Geometry check sheet. Reference: the model listing, model coordinates, mm. A direction names the side the tool comes from. Round coordinates to 2 decimals unless told otherwise and drop trailing zeros.
```python
from build123d import *

# Parameters (mm, degrees)
SKETCH1_R           = 2.5
BOSS_EXTRUDE1_DEPTH = 300
FILLET1_R           = 1.47
SKETCH2_R           = 1.5
CUT_EXTRUDE1_DEPTH  = 301.488285961
SKETCH3_R           = 1.5
CUT_EXTRUDE2_DEPTH  = 301.488286061
SKETCH4_R           = 1.5
CUT_EXTRUDE3_DEPTH  = 301.488286061


with BuildPart() as part:
    # Sketch1 → Boss-Extrude1 (new body)
    with BuildSketch(Plane.XY):
        Polygon((2.860553032, 3.9), (6, 7.039446968), (6, 8.2), (3.1, 8.2), (3.1, 10), (10, 10), (10, 3.1), (8.2, 3.1), (8.2, 6), (7.039446968, 6), (3.9, 2.860553032), (3.9, 0), (3.9, -2.860553032), (7.039446968, -6), (8.2, -6), (8.2, -3.1), (10, -3.1), (10, -10), (3.1, -10), (3.1, -8.2), (6, -8.2), (6, -7.039446968), (2.860553032, -3.9), (0, -3.9), (-2.860553032, -3.9), (-6, -7.039446968), (-6, -8.2), (-3.1, -8.2), (-3.1, -10), (-10, -10), (-10, -3.1), (-8.2, -3.1), (-8.2, -6), (-7.039446968, -6), (-3.9, -2.860553032), (-3.9, 0), (-3.9, 2.860553032), (-7.039446968, 6), (-8.2, 6), (-8.2, 3.1), (-10, 3.1), (-10, 10), (-3.1, 10), (-3.1, 8.2), (-6, 8.2), (-6, 7.039446968), (-2.860553032, 3.9), (0, 3.9), align=None)
        Circle(SKETCH1_R, mode=Mode.SUBTRACT)
    extrude(amount=BOSS_EXTRUDE1_DEPTH)

    # Fillet1
    fillet1_edges = [part.edges().sort_by_distance(p)[0] for p in [
        (10, -10, 150),
        (-10, -10, 150),
        (-10, 10, 150),
        (10, 10, 150),
    ]]
    fillet(fillet1_edges, radius=FILLET1_R)

    # Sketch2 → Cut-Extrude1 (cut, through all)
    with BuildSketch(Plane(origin=(3.9, 0, 0), x_dir=(0, 0, -1), z_dir=(1, 0, 0))):
        with Locations(Location((-150, 0, 0), (0, 0, 90))):
            Circle(SKETCH2_R)
    extrude(amount=-CUT_EXTRUDE1_DEPTH, mode=Mode.SUBTRACT)

    # Sketch3 → Cut-Extrude2 (cut, through all)
    with BuildSketch(Plane(origin=(3.9, 0, 0), x_dir=(0, 0, -1), z_dir=(1, 0, 0))):
        with Locations(Location((-77.5, 0, 0), (0, 0, 90))):
            Circle(SKETCH3_R)
    extrude(amount=-CUT_EXTRUDE2_DEPTH, mode=Mode.SUBTRACT)

    # Sketch4 → Cut-Extrude3 (cut, through all)
    with BuildSketch(Plane(origin=(0, 3.9, 0), x_dir=(1, 0, 0), z_dir=(0, 1, 0))):
        with Locations(Location((0, -50, 0), (0, 0, 180))):
            Circle(SKETCH4_R)
        with Locations(Location((0, -250, 0), (0, 0, 180))):
            Circle(SKETCH4_R)
    extrude(amount=-CUT_EXTRUDE3_DEPTH, mode=Mode.SUBTRACT)


solid = part.part
```
(1) Material ranges on line 1 (Z direction, x = -2.95, y = 0); line 2 (X direction, y = 5, z = 153); line 3 (Z direction, x = 0, y = 2.95), recorded low to high.
Returned:
line 1: z = 0 to 76, 79 to 148.5, 151.5 to 300
line 2: x = -10 to -8.2, -6.04 to -3.96, 3.96 to 6.04, 8.2 to 10
line 3: z = 0 to 48.5, 51.5 to 248.5, 251.5 to 300
(2) Set-up check for faces 1 (the flat face through (0, -3.9, 148)), 2 (the flat face through (3.9, 0, 148)), 3 (the flat face through (-3.9, 0, 148)), 4 (the flat face through (6, 10, 148)), 5 (the flat face through (-10, -6, 148)): record each of +Z, -Z, +X, -X, +Y, -Y from which the full face is reachable in a straight line by a thin tool's end or side.
Returned:
face 1: +Z, -Z, -Y
face 2: +Z, -Z, +X
face 3: +Z, -Z, -X
face 4: +Z, -Z, +X, -X, +Y
face 5: +Z, -Z, -X, +Y, -Y
(3) Draft check along X on faces 6 (the flat face through (10, 6, 148)), 7 (the flat face through (-2, 2, 0)), 8 (the flat face through (0, 3.9, 148)). Enter one of: released by +X, released by -X, zero draft, split by the parting line, or undercut.
Returned:
face 6: released by +X
face 7: zero draft
face 8: undercut
(4) Depth check by flat-ended pin: P1, Ø5, axis at x = 0, z = 50, coming from the +Y side; P2, Ø1.4, axis at x = 9.5, z = 198, coming from the -Y side (3 decimals); P3, Ø5, axis at y = 0, z = 77.5, coming from the +X side; P4, Ø2, axis at x = 6.5, y = -0.5, coming from the +Z side. Enter the tip coordinate at first touch or a pass-through.
Returned:
P1: stops at y = 3.9
P2: stops at y = -9.975
P3: stops at x = 3.9
P4: passes through
